from build123d import *

# Parameters (mm, degrees)
EXTRUDE_1_DEPTH      = 3
EXTRUDE_1_DEPTH_BACK = 3
EXTRUDE_2_DEPTH      = 4.5
EXTRUDE_2_DEPTH_BACK = 4.5
SKETCH_1_3_R         = 12
SKETCH_1_3_R_2       = 4.1
FILLET_1_R           = 2
FILLET_2_R           = 0.5
CUT_EXTRUDE_1_DEPTH  = 2


with BuildPart() as part:
    # 草图1 → 凸台-拉伸1 (new, two sides: drawn at the far end of the back side and taken through both)
    with BuildSketch(Plane.XY.offset(-EXTRUDE_1_DEPTH_BACK)):
        with BuildLine():
            Line((42.062746067, 9), (-42.062746067, 9))
            ThreePointArc((-42.062746067, 9), (-39.062746067, 4.937253933), (-38, 0))
            ThreePointArc((-38, 0), (-39.062746067, -4.937253933), (-42.062746067, -9))
            Line((-42.062746067, -9), (42.062746067, -9))
            ThreePointArc((42.062746067, -9), (38, 0), (42.062746067, 9))
        make_face()
    extrude(amount=EXTRUDE_1_DEPTH + EXTRUDE_1_DEPTH_BACK)

    # 草图1<3> → 凸台-拉伸2 (add, two sides: drawn at the far end of the back side and taken through both)
    # profile 1 of 2: a face of its own
    with BuildSketch(Plane.XY.offset(-EXTRUDE_2_DEPTH_BACK)):
        with Locations((-50, 0)):
            Circle(SKETCH_1_3_R)
        with Locations((-50, 0)):
            Circle(SKETCH_1_3_R_2, mode=Mode.SUBTRACT)
    # profile 2 of 2: a face of its own
    with BuildSketch(Plane.XY.offset(-EXTRUDE_2_DEPTH_BACK)):
        with Locations((50, 0)):
            Circle(SKETCH_1_3_R)
        with Locations((50, 0)):
            Circle(SKETCH_1_3_R_2, mode=Mode.SUBTRACT)
    extrude(amount=EXTRUDE_2_DEPTH + EXTRUDE_2_DEPTH_BACK)

    # 圆角1
    fillet_1_edges = [part.edges().sort_by_distance(p)[0] for p in [
        (42.062746067, -9, -1.5),
        (-42.062746067, -9, -1.5),
        (-42.062746067, 9, -1.5),
        (42.062746067, 9, -1.5),
    ]]
    fillet(fillet_1_edges, radius=FILLET_1_R)

    # 圆角2
    fillet_2_edges = [part.edges().sort_by_distance(p)[0] for p in [
        (-62, 0, -4.5),
        (-62, 0, 4.5),
        (38, 0, -4.5),
        (38, 0, 4.5),
    ]]
    fillet(fillet_2_edges, radius=FILLET_2_R)

    # 草图2 → 切除-拉伸1 (cut)
    with BuildSketch(Plane.XY.offset(3)):
        with BuildLine():
            Line((-28, 4), (28, 4))
            ThreePointArc((28, 4), (32, 0), (28, -4))
            Line((28, -4), (-28, -4))
            ThreePointArc((-28, -4), (-32, 0), (-28, 4))
        make_face()
    cut_extrude_1 = extrude(amount=-CUT_EXTRUDE_1_DEPTH, mode=Mode.SUBTRACT)

    # 镜向1: 切除-拉伸1 across plane
    add(cut_extrude_1.mirror(Plane.XY), mode=Mode.SUBTRACT)


solid = part.part
Read the model definition and answer for the solid it produces. Units are mm, in the model's axes. A direction names the side the tool comes from. Give positions to 0.01 mm unless a question says otherwise; leave off trailing zeros. Write each loop counter-clockwise with the first axis right and the second up, starting at its lowest first coordinate (ties: lowest second). Pieces come first, ordered by that corner, then holes. Notation, with made-up numbers: (46.25, -38.5) - (99.25, -38.5) arc R17 cw to (99.25, -31.5) - close; hole circle Ø11 at (69, 31.5). An arc over 180 degrees is marked (long way). Use CSV: the item, a comma, the result in double quotes. Start each with the question number.
(1) Given P1, Ø2, axis at x = 11.5, z = 1.5, coming from the -Y side; P2, Ø5.5, axis at x = -5, y = 0.5, coming from the -Z side; P3, Ø2, axis at x = 13.5, z = 2.5, coming from the +Y side, each flat-ended and moving along its own axis, determine where each tip first touches the part or whether it passes through.
(2) Find section A-A (x = -50). Give the vertices of the cut face in (y, z), plus the area to 3 significant figures.
(3) Find section C-C (x = 16.5). Give the vertices of the cut face in (y, z).
(4) Find section D-D (x = -36.5). Give the vertices of the cut face in (y, z).
(5) Determine the mould class of faces 5 (the flat face through (-0.6, 4.3, 3)), 6 (the flat face through (50, -5, 4.5)) for opening direction X: +X half, -X half, draft (parallel to the pull), parting line (faces both ways), or undercut.
(6) Consider line 1 along Y through (x, z) = (-9.5, 2.25); line 2 along Y through (x, z) = (50, 2.25); line 3 along X through (y, z) = (2.75, -3.75). Determine where each line is inside the solid, lowest interval first.
(7) Find section B-B (y = 0). Count the separate pieces of the cut face and the enclosed holes in it, plus the area to 3 significant figures.
(8) For faces 1 (the cylindrical face through (32, 0, 2)), 2 (the flat face through (-1, -9, 0)), 3 (the flat face through (1, 9, 0)), 4 (the flat face through (0, 0, -1)), determine the directions among +Z, -Z, +X, -X, +Y, -Y from which every point of the face is accessible in a straight line to the end or side of a thin tool.
Findings below:
1,P1,"y = -9"
1,P2,"z = -1"
1,P3,"y = 9"
2,outline,"(-12, -4) arc R0.5 ccw to (-11.5, -4.5) - (-4.1, -4.5) - (-4.1, 4.5) - (-11.5, 4.5) arc R0.5 ccw to (-12, 4) - close; (4.1, -4.5) - (11.5, -4.5) arc R0.5 ccw to (12, -4) - (12, 4) arc R0.5 ccw to (11.5, 4.5) - (4.1, 4.5) - close"
2,area,"142 mm2"
3,outline,"(-9, -3) - (-4, -3) - (-4, -1) - (4, -1) - (4, -3) - (9, -3) - (9, 3) - (4, 3) - (4, 1) - (-4, 1) - (-4, 3) - (-9, 3) - close"
4,outline,"(-9, -3) - (9, -3) - (9, 3) - (-9, 3) - close"
5,face 5,"undercut"
5,face 6,"draft"
6,line 1,"-9 to -4, 4 to 9"
6,line 2,"-12 to -4.1, 4.1 to 12"
6,line 3,"-61.68 to -53.04, -46.96 to -38.32, 38.32 to 46.96, 53.04 to 61.68"
7,separate pieces,"3"
7,enclosed holes,"0"
7,area,"484 mm2"
8,face 1,"+Z"
8,face 2,"+Z, -Z, -Y"
8,face 3,"+Z, -Z, +Y"
8,face 4,"-Z"
